The model under review builds one solid part; all positions refer to its coordinate system, in mm. A direction names the side the tool comes from. Round coordinates to 2 decimals unless told otherwise and drop trailing zeros. Order: outer loops, then holes, each group sorted by start corner. A loop starts at its lowest first (then second) coordinate and runs counter-clockwise, first axis right, second up.
1) Consider section A-A (z = 54). Give the boundary of the cut face in (x, y).
2) To check wall thickness, follow L1, parallel to X at y = -6.75, z = 47.5; L2, parallel to Y at x = 7.5, z = 45.5; L3, parallel to Z at x = -18.5, y = -16. State the ranges of each line that lie inside material, in increasing order.
3) Consider section D-D (y = -20). Give the boundary of the cut face in (x, z), then the cut area to 3 significant figures.
4) Consider section C-C (z = 28). Give the boundary of the cut face in (x, y), then the cut area to 3 significant figures.
5) Consider section B-B (y = -16). Give the boundary of the cut face in (x, z).
6) Machinability: for faces 5 (the face through (0, -1.5, 30)), 6 (the face through (-2, -1, 57)), 7 (the face through (0, -1, 0)), which of the approach directions +Z, -Z, +X, -X, +Y, -Y give a long, thin tool a straight path to every point of the face, cutting with its end or side? Answer none if there is none.
7) Clearance check with flat-ended pins moving along their axes: P1, Ø4, axis at x = -13, z = 53.5, coming from the -Y side; P2, Ø0.8, axis at y = -0.5, z = 57.5, coming from the -X side; P3, Ø1.6, axis at y = -0.5, z = 58, coming from the +X side. State where each tip first meets the part, or that it passes through.
8) Mouldability with a two-part tool opening along X and no side actions: class faces 1 (the face through (-19.2, -10, 37)), 2 (the face through (18.53, -0.64, 30.42)), 3 (the face through (18, -16, 56)), 4 (the face through (17.7, -10, 37)) as pulls with the +X half, pulls with the -X half, needs draft (parallel to the pull), parting line crosses it, or undercut.
from build123d import *

# Parameters (mm, degrees)
SKETCH1_W                    = 17.7
SKETCH1_H                    = 60
BASE_FLANGE2_DEPTH           = 1.5
EDGE_FLANGE2_STRIP_W         = 7.4732
EDGE_FLANGE2_STRIP_H         = 1.5
EDGE_FLANGE2_STRIP_CUT_DEPTH = 60
EDGE_FLANGE2_DEPTH           = 60
CUT_EXTRUDE5_DEPTH           = 1.5
FILLET4_R                    = 5
FILLET5_R                    = 3
SKETCH22_R                   = 2
CUT_EXTRUDE6_DEPTH           = 1.5
CUT_EXTRUDE7_REACH           = 68.728
FILLET6_R                    = 1


# Sheet-metal steps are written as plain solids
with BuildPart() as part:
    # Sketch1 → Base-Flange2 (new body)
    with BuildSketch(Plane(origin=(0, 0, 0), x_dir=(1, 0, 0), z_dir=(0, 1, 0))):
        with Locations((-8.85, -30)):
            Rectangle(SKETCH1_W, SKETCH1_H)
    extrude(amount=-BASE_FLANGE2_DEPTH)

    # Edge-Flange2 strip (across the edge) → Edge-Flange2 strip cut (cut)
    with BuildSketch(Plane(origin=(-17.7, -1.5, 60), x_dir=(1, 0, 0), z_dir=(0, 0, -1))):
        with Locations((-3, -0.75)):
            Rectangle(EDGE_FLANGE2_STRIP_W, EDGE_FLANGE2_STRIP_H)
    extrude(amount=EDGE_FLANGE2_STRIP_CUT_DEPTH, mode=Mode.SUBTRACT)

    # Edge-Flange2 section (across the edge) → Edge-Flange2 (add)
    with BuildSketch(Plane(origin=(-17.7, -1.5, 60), x_dir=(1, 0, 0), z_dir=(0, 0, -1))):
        with BuildLine():
            Line((-1.5, 0.7366), (-1.5, 20.5))
            Line((-1.5, 20.5), (0, 20.5))
            Line((0, 20.5), (0, 0.7366))
            ThreePointArc((0, 0.7366), (0.215745145, 0.215745145), (0.7366, 0))
            Line((0.7366, 0), (0.7366, -1.5))
            ThreePointArc((0.7366, -1.5), (-0.844915027, -0.844915027), (-1.5, 0.7366))
        make_face()
    extrude(amount=EDGE_FLANGE2_DEPTH)

    # Sketch20 → Cut-Extrude5 (cut)
    with BuildSketch(Plane.ZY.offset(19.2)):
        Polygon((0, -5), (40, -22), (0, -22), align=None)
    extrude(amount=-CUT_EXTRUDE5_DEPTH, mode=Mode.SUBTRACT)

    # Fillet4
    fillet4_edges = [part.edges().sort_by_distance(p)[0] for p in [
        (-18.45, -22, 60),
        (-18.45, -22, 40),
    ]]
    fillet(fillet4_edges, radius=FILLET4_R)

    # Fillet5
    fillet5_edges = [part.edges().sort_by_distance(p)[0] for p in [
        (-18.45, -5, 0),
    ]]
    fillet(fillet5_edges, radius=FILLET5_R)

    # Sketch22 → Cut-Extrude6 (cut)
    with BuildSketch(Plane.ZY.offset(19.2)):
        with Locations(Location((54, -16, 0), (0, 0, 270))):
            Circle(SKETCH22_R)
    extrude(amount=-CUT_EXTRUDE6_DEPTH, mode=Mode.SUBTRACT)

    # Mirror1: part across plane


with BuildPart() as part_1:
    add(part.part)
    add(part.part.mirror(Plane(origin=(0, -1.5, 60), x_dir=(0, 0, 1), z_dir=(1, 0, 0))))

    # Sketch28 → Cut-Extrude7 (cut, up to next)
    with BuildSketch(Plane(origin=(0, 0, 0), x_dir=(1, 0, 0), z_dir=(0, 1, 0)), mode=Mode.PRIVATE) as cut_extrude7_sk1:
        with BuildLine():
            Line((2, -55), (2, -60))
            Line((2, -60), (-2, -60))
            Line((-2, -60), (-2, -55))
            ThreePointArc((-2, -55), (0, -53), (2, -55))
        make_face()
    cut_extrude7_tool1 = extrude(cut_extrude7_sk1.sketch, amount=-CUT_EXTRUDE7_REACH, mode=Mode.PRIVATE) & part_1.part
    add(cut_extrude7_tool1.solids().sort_by_distance((0, 0, 56.699439))[0], mode=Mode.SUBTRACT)

    # Fillet6
    fillet6_edges = [part_1.edges().sort_by_distance(p)[0] for p in [
        (2, -0.75, 60),
        (-2, -0.75, 60),
    ]]
    fillet(fillet6_edges, radius=FILLET6_R)


solid = part_1.part
Answer below:
1. outline: (-19.2, -22) - (-17.7, -22) - (-17.7, -18) - (-19.2, -18) - close; (-19.2, -14) - (-17.7, -14) - (-17.7, -2.24) arc R0.74 cw to (-16.96, -1.5) - (-1.73, -1.5) - (-1.73, 0) - (-16.96, 0) arc R2.24 ccw to (-19.2, -2.24) - close; (1.73, -1.5) - (16.96, -1.5) arc R0.74 cw to (17.7, -2.24) - (17.7, -14) - (19.2, -14) - (19.2, -2.24) arc R2.24 ccw to (16.96, 0) - (1.73, 0) - close; (17.7, -22) - (19.2, -22) - (19.2, -18) - (17.7, -18) - close
2. L1: x = -19.2 to -17.7, 17.7 to 19.2
2. L2: y = -1.5 to 0
2. L3: z = 25.88 to 52, 56 to 60
3. outline: (-19.2, 35.29) - (-17.7, 35.29) - (-17.7, 59) - (-19.2, 59) - close; (17.7, 35.29) - (19.2, 35.29) - (19.2, 59) - (17.7, 59) - close
3. area: 71.1 mm2
4. outline: (-19.2, -16.9) - (-17.7, -16.9) - (-17.7, -2.24) arc R0.74 cw to (-16.96, -1.5) - (16.96, -1.5) arc R0.74 cw to (17.7, -2.24) - (17.7, -16.9) - (19.2, -16.9) - (19.2, -2.24) arc R2.24 ccw to (16.96, 0) - (-16.96, 0) arc R2.24 ccw to (-19.2, -2.24) - close
4. area: 102 mm2
5. outline: (-19.2, 25.88) - (-17.7, 25.88) - (-17.7, 52) - (-19.2, 52) - close; (-19.2, 56) - (-17.7, 56) - (-17.7, 60) - (-19.2, 60) - close; (17.7, 25.88) - (19.2, 25.88) - (19.2, 52) - (17.7, 52) - close; (17.7, 56) - (19.2, 56) - (19.2, 60) - (17.7, 60) - close
6. face 5: +Z, -Z, -Y
6. face 6: +Z, +Y, -Y
6. face 7: -Z, +X, -X, +Y, -Y
7. P1: stops at y = -1.5
7. P2: stops at x = -18.76
7. P3: stops at x = 18.99
8. face 1: pulls with the -X half
8. face 2: pulls with the +X half
8. face 3: needs draft
8. face 4: undercut
